Geometry check sheet. Reference: the model listing, model coordinates, mm. A direction names the side the tool comes from. Round coordinates to 2 decimals unless told otherwise and drop trailing zeros. Write each loop counter-clockwise with the first axis right and the second up, starting at its lowest first coordinate (ties: lowest second). Pieces come first, ordered by that corner, then holes.
Item 1: Scan lines: probe 1 along Z at (x, y) = (4, 1.95); probe 2 along Y at (x, z) = (12.5, 19); probe 3 along X at (y, z) = (3.1, 22). Record each from-to range of solid material in increasing order.
Item 2: Cross-section at B-B (y = 1.5). Enter the section's corners in (x, z), then the cut area to 3 significant figures.
Item 3: Depth check by flat-ended pin: P1, Ø0.8, axis at y = 1, z = 9.5, coming from the -X side; P2, Ø3, axis at x = 11.5, z = 21, coming from the +Y side. Enter the tip coordinate at first touch or a pass-through.
Item 4: Cross-section at D-D (x = 36.5). Enter the section's corners in (y, z), then the cut area to 3 significant figures.
Item 5: Access from +Z, -Z, +X, -X, +Y, -Y to the whole of each face (thin tool, end or side, straight path). Record for faces 4 (the face through (15, 1, 24)), 5 (the face through (3.254, 2.392, 16.409)).
Item 6: Draft check along Z on faces 1 (the face through (25, 1, 0)), 2 (the face through (15, 1, 23)), 3 (the face through (0, 1, 29)). Enter one of: pulls with the +Z half, pulls with the -Z half, needs draft (parallel to the pull), parting line crosses it, or undercut.
Item 7: Cross-section at C-C (z = 2). Enter the section's corners in (x, y).
Item 8: Cross-section at A-A (x = 29.5). Enter the section's corners in (y, z), then the cut area to 3 significant figures.
from build123d import *

# Parameters (mm, degrees)
SKETCH2_W           = 33
SKETCH2_H           = 2
BOSS_EXTRUDE1_DEPTH = 50
SKETCH3_W           = 30
SKETCH3_H           = 1
CUT_EXTRUDE2_DEPTH  = 50
SKETCH4_W           = 3
SKETCH4_H           = 13
BOSS_EXTRUDE2_DEPTH = 2
CUT_EXTRUDE3_DEPTH  = 13
FILLET1_R           = 10
FILLET2_R           = 0.5


with BuildPart() as part:
    # Sketch2 → Boss-Extrude1 (new body)
    with BuildSketch(Plane(origin=(0, 0, 0), x_dir=(0, 0, -1), z_dir=(1, 0, 0))):
        with Locations((-16.5, 1)):
            Rectangle(SKETCH2_W, SKETCH2_H)
    extrude(amount=BOSS_EXTRUDE1_DEPTH)

    # Sketch3 → Cut-Extrude2 (cut)
    with BuildSketch(Plane(origin=(0, 2, 0), x_dir=(1, 0, 0), z_dir=(0, 1, 0))):
        with Locations((15, -9.5)):
            Rectangle(SKETCH3_W, SKETCH3_H)
        with Locations((15, -23.5)):
            Rectangle(SKETCH3_W, SKETCH3_H)
    extrude(amount=-CUT_EXTRUDE2_DEPTH, mode=Mode.SUBTRACT)

    # Sketch4 → Boss-Extrude2 (add)
    with BuildSketch(Plane(origin=(0, 2, 0), x_dir=(1, 0, 0), z_dir=(0, 1, 0))):
        with Locations((1.5, -16.5)):
            Rectangle(SKETCH4_W, SKETCH4_H)
    extrude(amount=BOSS_EXTRUDE2_DEPTH)

    # Sketch5 → Cut-Extrude3 (cut)
    with BuildSketch(Plane.XY.offset(23)):
        Polygon((3, 2), (0, 4), (3, 4), align=None)
    extrude(amount=-CUT_EXTRUDE3_DEPTH, mode=Mode.SUBTRACT)

    # Fillet1
    fillet1_edges = [part.edges().sort_by_distance(p)[0] for p in [
        (3, 2, 16.5),
    ]]
    fillet(fillet1_edges, radius=FILLET1_R)

    # Fillet2
    fillet2_edges = [part.edges().sort_by_distance(p)[0] for p in [
        (0, 4, 16.5),
    ]]
    fillet(fillet2_edges, radius=FILLET2_R)


solid = part.part
Resolved:
1. probe 1: z = 0 to 9, 10 to 23, 24 to 33
1. probe 2: y = 0 to 2
1. probe 3: x = 0 to 1.47
2. outline: (0, 0) - (50, 0) - (50, 33) - (0, 33) - (0, 24) - (30, 24) - (30, 23) - (0, 23) - (0, 10) - (30, 10) - (30, 9) - (0, 9) - close
2. area: 1,590 mm2
3. P1: stops at x = 30
3. P2: stops at y = 2
4. outline: (0, 0) - (2, 0) - (2, 33) - (0, 33) - close
4. area: 66.0 mm2
5. face 4: -X, +Y, -Y
5. face 5: +Z, -Z, +X, +Y
6. face 1: pulls with the -Z half
6. face 2: undercut
6. face 3: needs draft
7. outline: (0, 0) - (50, 0) - (50, 2) - (0, 2) - close
8. outline: (0, 0) - (2, 0) - (2, 9) - (0, 9) - close; (0, 10) - (2, 10) - (2, 23) - (0, 23) - close; (0, 24) - (2, 24) - (2, 33) - (0, 33) - close
8. area: 62.0 mm2
